```python
from build123d import *

# Parameters (mm, degrees)
SKETCH_1_W             = 23.5
SKETCH_1_H             = 12
EXTRUDE_1_DEPTH        = 175
HOLE_WIZARD_M6_1_D     = 5
HOLE_WIZARD_M6_1_DEPTH = 15
HOLE_WIZARD_M6_1_TIP   = 1.502151548
HOLE_WIZARD_M6_2_D     = 5
HOLE_WIZARD_M6_2_DEPTH = 15
HOLE_WIZARD_M6_2_TIP   = 1.502151548
HOLE_WIZARD_M4_1_D     = 3.3
HOLE_WIZARD_M4_1_DEPTH = 10.1
HOLE_WIZARD_M4_1_TIP   = 0.991420021
HOLE_WIZARD_M6_3_D     = 5
HOLE_WIZARD_M6_3_DEPTH = 15
HOLE_WIZARD_M6_3_TIP   = 1.502151548


with BuildPart() as part:
    # 草图1 → 凸台-拉伸1 (new, symmetric)
    with BuildSketch(Plane(origin=(0, 0, 0), x_dir=(0, 0, -1), z_dir=(1, 0, 0))):
        with BuildLine():
            Line((-14, 15), (-11.5, 15))
            Line((-11.5, 15), (-11.5, 13.5))
            Line((-11.5, 13.5), (-11.4, 13.5))
            ThreePointArc((-11.4, 13.5), (-11.117157288, 13.382842712), (-11, 13.1))
            Line((-11, 13.1), (-11, 12))
            Line((-11, 12), (-9.5, 12))
            Line((-9.5, 12), (-9.5, 15))
            Line((-9.5, 15), (-8, 15))
            Line((-8, 15), (-8, 12.5))
            Line((-8, 12.5), (-5, 12.5))
            Line((-5, 12.5), (-5, 15))
            Line((-5, 15), (5, 15))
            Line((5, 15), (5, 12.5))
            Line((5, 12.5), (8, 12.5))
            Line((8, 12.5), (8, 15))
            Line((8, 15), (9.5, 15))
            Line((9.5, 15), (9.5, 12))
            Line((9.5, 12), (11, 12))
            Line((11, 12), (11, 13.1))
            ThreePointArc((11, 13.1), (11.117157288, 13.382842712), (11.4, 13.5))
            Line((11.4, 13.5), (11.5, 13.5))
            Line((11.5, 13.5), (11.5, 15))
            Line((11.5, 15), (14, 15))
            ThreePointArc((14, 15), (14.707106781, 14.707106781), (15, 14))
            Line((15, 14), (15, 8))
            Line((15, 8), (12.5, 8))
            Line((12.5, 8), (12.5, 5))
            Line((12.5, 5), (15, 5))
            Line((15, 5), (15, -5))
            Line((15, -5), (12.5, -5))
            Line((12.5, -5), (12.5, -8))
            Line((12.5, -8), (15, -8))
            Line((15, -8), (15, -14))
            ThreePointArc((15, -14), (14.707106781, -14.707106781), (14, -15))
            Line((14, -15), (11.5, -15))
            Line((11.5, -15), (11.5, -13.5))
            Line((11.5, -13.5), (11.4, -13.5))
            ThreePointArc((11.4, -13.5), (11.117157288, -13.382842712), (11, -13.1))
            Line((11, -13.1), (11, -12))
            Line((11, -12), (9.5, -12))
            Line((9.5, -12), (9.5, -15))
            Line((9.5, -15), (8, -15))
            Line((8, -15), (8, -12.5))
            Line((8, -12.5), (5, -12.5))
            Line((5, -12.5), (5, -15))
            Line((5, -15), (-5, -15))
            Line((-5, -15), (-5, -12.5))
            Line((-5, -12.5), (-8, -12.5))
            Line((-8, -12.5), (-8, -15))
            Line((-8, -15), (-9.5, -15))
            Line((-9.5, -15), (-9.5, -12))
            Line((-9.5, -12), (-11, -12))
            Line((-11, -12), (-11, -13.1))
            ThreePointArc((-11, -13.1), (-11.117157288, -13.382842712), (-11.4, -13.5))
            Line((-11.4, -13.5), (-11.5, -13.5))
            Line((-11.5, -13.5), (-11.5, -15))
            Line((-11.5, -15), (-14, -15))
            ThreePointArc((-14, -15), (-14.707106781, -14.707106781), (-15, -14))
            Line((-15, -14), (-15, 14))
            ThreePointArc((-15, 14), (-14.707106781, 14.707106781), (-14, 15))
        make_face()
        with BuildLine():
            Line((12, -10.5), (12, -8.5))
            ThreePointArc((12, -8.5), (11.853553391, -8.146446609), (11.5, -8))
            Line((11.5, -8), (-11.5, -8))
            ThreePointArc((-11.5, -8), (-11.853553391, -8.146446609), (-12, -8.5))
            Line((-12, -8.5), (-12, -10.5))
            ThreePointArc((-12, -10.5), (-11.853553391, -10.853553391), (-11.5, -11))
            Line((-11.5, -11), (11.5, -11))
            ThreePointArc((11.5, -11), (11.853553391, -10.853553391), (12, -10.5))
        make_face(mode=Mode.SUBTRACT)
        with BuildLine():
            Line((-11.5, 11), (11.5, 11))
            ThreePointArc((11.5, 11), (11.853553391, 10.853553391), (12, 10.5))
            Line((12, 10.5), (12, 8.5))
            ThreePointArc((12, 8.5), (11.853553391, 8.146446609), (11.5, 8))
            Line((11.5, 8), (-11.5, 8))
            ThreePointArc((-11.5, 8), (-11.853553391, 8.146446609), (-12, 8.5))
            Line((-12, 8.5), (-12, 10.5))
            ThreePointArc((-12, 10.5), (-11.853553391, 10.853553391), (-11.5, 11))
        make_face(mode=Mode.SUBTRACT)
        Rectangle(SKETCH_1_W, SKETCH_1_H, mode=Mode.SUBTRACT)
    extrude(amount=EXTRUDE_1_DEPTH, both=True)

    # M6 螺纹孔1
    with Locations(Plane(origin=(0, 15, 0), x_dir=(-1, 0, 0), z_dir=(0, 1, 0))):
        with Locations((-155, 0), (-140, 0), (140, 0), (155, 0)):
            Hole(HOLE_WIZARD_M6_1_D / 2, depth=HOLE_WIZARD_M6_1_DEPTH)
            with Locations((0, 0, -(HOLE_WIZARD_M6_1_DEPTH + HOLE_WIZARD_M6_1_TIP / 2))):  # 118° drill point
                Cone(0, HOLE_WIZARD_M6_1_D / 2, HOLE_WIZARD_M6_1_TIP, mode=Mode.SUBTRACT)

    # M6 螺纹孔2
    with Locations(Plane.XZ.offset(15)):
        with Locations((155, 0), (140, 0), (-140, 0), (-155, 0)):
            Hole(HOLE_WIZARD_M6_2_D / 2, depth=HOLE_WIZARD_M6_2_DEPTH)
            with Locations((0, 0, -(HOLE_WIZARD_M6_2_DEPTH + HOLE_WIZARD_M6_2_TIP / 2))):  # 118° drill point
                Cone(0, HOLE_WIZARD_M6_2_D / 2, HOLE_WIZARD_M6_2_TIP, mode=Mode.SUBTRACT)

    # M4 螺纹孔1
    with Locations(Plane(origin=(0, 0, -15), x_dir=(-1, 0, 0), z_dir=(0, 0, -1))):
        with Locations((145, 0), (45, 0), (-55, 0)):
            Hole(HOLE_WIZARD_M4_1_D / 2, depth=HOLE_WIZARD_M4_1_DEPTH)
            with Locations((0, 0, -(HOLE_WIZARD_M4_1_DEPTH + HOLE_WIZARD_M4_1_TIP / 2))):  # 118° drill point
                Cone(0, HOLE_WIZARD_M4_1_D / 2, HOLE_WIZARD_M4_1_TIP, mode=Mode.SUBTRACT)

    # M6 螺纹孔3
    with Locations(Plane(origin=(0, 15, 0), x_dir=(-1, 0, 0), z_dir=(0, 1, 0))):
        with Locations((105, 0), (-105, 0)):
            Hole(HOLE_WIZARD_M6_3_D / 2, depth=HOLE_WIZARD_M6_3_DEPTH)
            with Locations((0, 0, -(HOLE_WIZARD_M6_3_DEPTH + HOLE_WIZARD_M6_3_TIP / 2))):  # 118° drill point
                Cone(0, HOLE_WIZARD_M6_3_D / 2, HOLE_WIZARD_M6_3_TIP, mode=Mode.SUBTRACT)


solid = part.part
```
Geometry check sheet. Reference: the model listing, model coordinates, mm. A direction names the side the tool comes from. Give positions to 0.01 mm unless a question says otherwise; leave off trailing zeros.
1) Access from +Z, -Z, +X, -X, +Y, -Y to the whole of each face (thin tool, end or side, straight path). Record for faces 1 (the flat face through (2, 8, 0)), 2 (the flat face through (175, 7, 0)).
2) Gauge pin test, flat ends, axial feed: pin 1 (4.5 mm diameter, centred on x = 155, z = 0, fed in from +Y); pin 2 (6 mm diameter, centred on x = -155, z = 0, fed in from +Y). Record the tip position at first contact, or that the pin passes through.
3) Section check A-A, the plane x = 125. State how many separate pieces and enclosed holes the cut face has, and give its area (3 significant figures).
4) Material ranges on L1, parallel to Y at x = -68, z = 2.25; L2, parallel to Y at x = 83.5, z = 6; L3, parallel to Z at x = 155, y = -13.3, recorded low to high.
5) Release check for a two-part mould opening along Z. For faces 3 (the flat face through (2, -8, 0)), 4 (the flat face through (2, 15, 0)), 5 (the flat face through (2, 0, 15)) record: pulls with the +Z half, pulls with the -Z half, needs draft (parallel to the pull), parting line crosses it, or undercut.
Computed:
1. face 1: +X, -X
1. face 2: +Z, -Z, +X, +Y, -Y
2. pin 1: passes through
2. pin 2: stops at y = 15
3. separate pieces: 1
3. enclosed holes: 3
3. area: 407 mm2
4. L1: y = -15 to -11, -8 to -6, 6 to 8, 11 to 15
4. L2: y = -12.5 to -11, -8 to -6, 6 to 8, 11 to 12.5
4. L3: z = -15 to -11.05, -9.5 to -8, -5 to -2.5, 2.5 to 5, 8 to 9.5, 11.05 to 15
5. face 3: undercut
5. face 4: needs draft
5. face 5: pulls with the +Z half
